from build123d import *

# Parameters (mm, degrees)
BOSS_EXTRUDE1_DEPTH   = 3.175
BOSS_EXTRUDE2_DEPTH   = 3.175
F_4_CLEARANCE_HOLE1_D = 2.9464


with BuildPart() as part:
    # Sketch1 → Boss-Extrude1 (new body)
    with BuildSketch(Plane(origin=(0, 0, -14.15699402), x_dir=(-1, 0, 0), z_dir=(0, 0, -1))):
        with BuildLine():
            Line((-49.172312317, -34.502108483), (-53.141062317, -27.628031841))
            ThreePointArc((-53.141062317, -27.628031841), (-55.063803638, -24.012221257), (-56.72992661, -20.271224785))
            ThreePointArc((-56.72992661, -20.271224785), (-54.976138042, -16.13776671), (-50.842679967, -17.891555277))
            ThreePointArc((-50.842679967, -17.891555277), (-49.356678398, -21.228119699), (-47.641801003, -24.453031841))
            Line((-47.641801003, -24.453031841), (-43.673051003, -31.327108483))
            ThreePointArc((-43.673051003, -31.327108483), (-16.68272836, -52.037511462), (17.046778195, -47.596937682))
            Line((17.046778195, -47.596937682), (23.920854837, -43.628187682))
            Line((23.920854837, -43.628187682), (30.79493148, -39.659437682))
            ThreePointArc((30.79493148, -39.659437682), (51.505334458, -12.669115038), (47.064760678, 21.060391517))
            Line((47.064760678, 21.060391517), (43.096010678, 27.934468159))
            ThreePointArc((43.096010678, 27.934468159), (41.160593535, 31.032051618), (39.01404477, 33.987248938))
            ThreePointArc((39.01404477, 33.987248938), (39.561948355, 38.44382292), (44.018522337, 37.895919335))
            ThreePointArc((44.018522337, 37.895919335), (46.425258832, 34.58251628), (48.595271992, 31.109468159))
            Line((48.595271992, 31.109468159), (52.564021992, 24.235391517))
            ThreePointArc((52.564021992, 24.235391517), (57.638963455, -14.312615975), (33.96993148, -45.158698996))
            Line((33.96993148, -45.158698996), (27.095854837, -49.127448996))
            Line((27.095854837, -49.127448996), (20.221778195, -53.096198996))
            ThreePointArc((20.221778195, -53.096198996), (-18.326229296, -58.171140459), (-49.172312317, -34.502108483))
        make_face()
    extrude(amount=BOSS_EXTRUDE1_DEPTH)

    # Sketch6 → Boss-Extrude2 (add)
    with BuildSketch(Plane.XY.offset(-14.15699402)):
        Polygon((82.197110068, -48.248224024), (61.788603461, -72.570135093), (31.367040987, -47.043413242), (51.775547595, -22.721502173), align=None)
        with BuildLine():
            Line((64.875367382, -39.847664977), (67.930199412, -42.410973407))
            ThreePointArc((67.930199412, -42.410973407), (69.307717782, -58.156080429), (53.56261076, -59.533598799))
            Line((53.56261076, -59.533598799), (50.50777873, -56.970290369))
            ThreePointArc((50.50777873, -56.970290369), (49.130260359, -41.225183347), (64.875367382, -39.847664977))
        make_face(mode=Mode.SUBTRACT)
        with BuildLine():
            Line((61.233994962, -68.291668614), (58.179162931, -65.728360184))
            ThreePointArc((58.179162931, -65.728360184), (58.000711688, -63.688653138), (60.040418734, -63.510201894))
            Line((60.040418734, -63.510201894), (63.095250764, -66.073510324))
            ThreePointArc((63.095250764, -66.073510324), (63.273702008, -68.11321737), (61.233994962, -68.291668614))
        make_face(mode=Mode.SUBTRACT)
        with BuildLine():
            Line((42.411897591, -48.718116305), (45.466729621, -51.281424735))
            ThreePointArc((45.466729621, -51.281424735), (45.645180865, -53.321131781), (43.605473819, -53.499583025))
            Line((43.605473819, -53.499583025), (40.550641788, -50.936274595))
            ThreePointArc((40.550641788, -50.936274595), (40.372190545, -48.896567549), (42.411897591, -48.718116305))
        make_face(mode=Mode.SUBTRACT)
        with BuildLine():
            Line((57.20398318, -31.089595162), (60.25881521, -33.652903592))
            ThreePointArc((60.25881521, -33.652903592), (60.437266454, -35.692610638), (58.397559408, -35.871061882))
            Line((58.397559408, -35.871061882), (55.342727378, -33.307753452))
            ThreePointArc((55.342727378, -33.307753452), (55.164276134, -31.268046406), (57.20398318, -31.089595162))
        make_face(mode=Mode.SUBTRACT)
        with BuildLine():
            Line((74.832504323, -45.881680752), (77.887336353, -48.444989181))
            ThreePointArc((77.887336353, -48.444989181), (78.065787597, -50.484696227), (76.026080551, -50.663147471))
            Line((76.026080551, -50.663147471), (72.97124852, -48.099839041))
            ThreePointArc((72.97124852, -48.099839041), (72.792797277, -46.060131995), (74.832504323, -45.881680752))
        make_face(mode=Mode.SUBTRACT)
    extrude(amount=-BOSS_EXTRUDE2_DEPTH)

    # #4 Clearance Hole1 (through all)
    with Locations(Plane(origin=(0, 0, -17.33199402), x_dir=(-1, 0, 0), z_dir=(0, 0, -1))):
        with Locations((-53.56643166, -20.541270527), (-47.21643166, -31.539793155), (42.670641335, 35.021229473), (49.020641335, 24.022706845)):
            Hole(F_4_CLEARANCE_HOLE1_D / 2)


solid = part.part
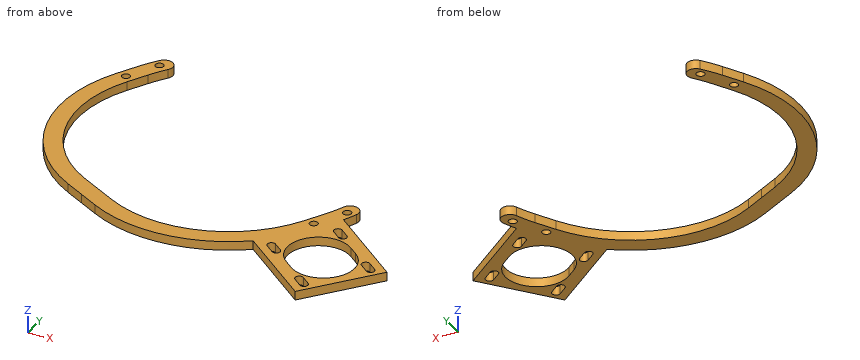
The model under review builds one solid part; all positions refer to its coordinate system, in mm. Coordinates: 2 decimals unless noted, no trailing zeros. Order: outer loops, then holes, each group sorted by start corner. A loop starts at its lowest first (then second) coordinate and runs counter-clockwise, first axis right, second up. Notation, with made-up numbers: (45.5, 65.5) -> (74.5, 65.5) arc R33 cw to (74.5, 95.5) -> close; hole circle Ø10 at (50, 9.25). An arc over 180 degrees is marked (long way). Answer in a Markdown table with one row per item.
(1) Consider section B-B (z = -16.5). State how many separate pieces and enclosed holes the cut face has, plus the area to 3 significant figures.
Answers:
| item | result |
|---|---|
| separate pieces | 1 |
| enclosed holes | 9 |
| area | 1,790 mm² |
(2) Wall thickness on line 1 along Y through (x, z) = (43, -14.5); line 2 along X through (y, z) = (-34, -16.45); line 3 along X through (y, z) = (34, -16.9): over which ranges is each line inside the solid? List them lowest first.
Answers:
| item | result |
|---|---|
| line 1 | -56.8 to -52.99, -49.21 to -32.45 |
| line 2 | -47.33 to -38.53, 42 to 56.17, 60.56 to 65.22 |
| line 3 | -46.81 to -43.73, -41.61 to -39 |
(3) Consider section C-C (x = 0.5). Write out the cut boundary in (y, z).
Answers:
| item | result |
|---|---|
| outline | (-59.69, -17.33) -> (-53.31, -17.33) -> (-53.31, -14.16) -> (-59.69, -14.16) -> close |
(4) Insertion check: pin 1 (1 mm diameter, centred on y = -20.5, z = -16, fed in from -X); pin 2 (1 mm diameter, centred on x = 60, z = -16.5, fed in from -Y); pin 3 (3.5 mm diameter, centred on x = 53.57, y = -20.54, fed in from +Z); pin 4 (1.5 mm diameter, centred on y = -26, z = -16.5, fed in from -X). Each pin has a flat end and moves straight along its axis. Give the tip position at first contact, or say it passes through.
Answers:
| item | result |
|---|---|
| pin 1 | x = -55.75 |
| pin 2 | y = -71.49 |
| pin 3 | z = -14.16 |
| pin 4 | x = -53.3 |
(5) Consider section A-A (y = 10). Write out the cut boundary in (x, z).
Answers:
| item | result |
|---|---|
| outline | (-58.13, -17.33) -> (-51.59, -17.33) -> (-51.59, -14.16) -> (-58.13, -14.16) -> close |
